Autodesk Inventor part; units mm, degrees
ref_plane "YZ Plane" through (0, 0, 0) normal (1, 0, 0) x (0, 1, 0)
ref_plane "XZ Plane" through (0, 0, 0) normal (0, 1, 0) x (-1, 0, 0)
ref_plane "XY Plane" through (0, 0, 0) normal (0, 0, 1) x (1, 0, 0)
sketch "Skizze1" plane through (0, 0, 0) normal (1, 0, 0) x (0, 1, 0)
  line L0 (0, 0) -> (-10, 0) construction
  circle A0 centre (0, 0) radius 1.1
  circle A1 centre (-10, 0) radius 1.1
  arc A2 (-10, 2.5) -> (-10, -2.5) centre (-10, 0) ccw
  line L1 (-10, -2.5) -> (1.8, -2.5)
  line L2 (-10, 2.5) -> (-0.7, 2.5)
  arc A3 (1.8, 0) -> (-0.7, 2.5) centre (-0.7, 0) ccw
  line L3 (1.8, 0) -> (1.8, -2.5)
  dimension "d0" = 10
  dimension "d1" = 2.2
  dimension "d2" = 2.2
  dimension "d3" = 2.5
  dimension "d8" = 2.5
  dimension "d9" = 1.8
extrude "Extrusion1" add sketch "Skizze1" along normal mid plane 4
chamfer "Fase1" distance 0.5 angle 45 10 edges at (2, 1.0678, 1.7678) (2, -5.35, 2.5) (2, -12.5, 0) (2, -4.1, -2.5) (2, 1.8, -1.25) (-2, 1.0678, 1.7678) (-2, -5.35, 2.5) (-2, -12.5, 0) (-2, -4.1, -2.5) (-2, 1.8, -1.25)
sketch "Skizze5" plane through (-1.5, -10, 2.5) normal (0, 0, 1) x (1, 0, 0)
  line L0 (1.5, 14.66) -> (1.5, -5.36)
  line L1 (-1.3, 10) -> (4.3, 10)
  line L2 (3.5, 8) -> (-0.5, 8)
  line L3 (-0.5, 8) -> (-0.5, 7)
  line L4 (-0.5, 7) -> (3.5, 7)
  line L5 (3.5, 7) -> (3.5, 8)
  line L6 (3.5, 0) -> (3.5, 9.3)
  line L7 (-0.5, 9.3) -> (-0.5, 0)
  point P0 (1.5, 10)
  dimension "d26" = 1
  dimension "d27" = 2
extrude "Extrusion4" cut sketch "Skizze5" against normal blind 1
equation "\"d2\" = d1"
properties part number "Chipanschlag TN1"
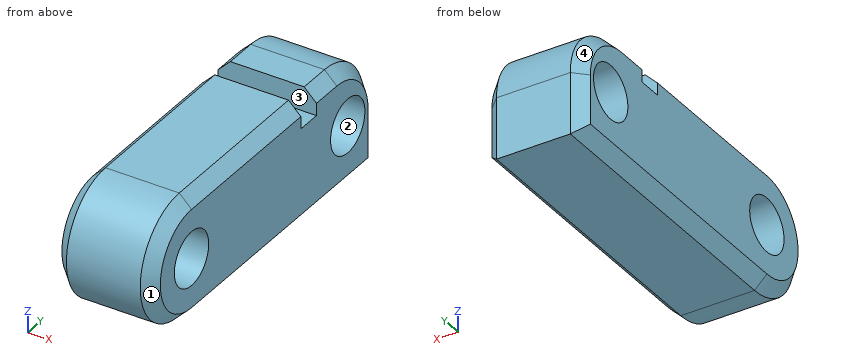
Part model, mm, in its own coordinate system. Face numbers are marked on the shaded views. Round coordinates to 2 decimals unless told otherwise and drop trailing zeros. Loops run counter-clockwise (first coordinate to the right, second up) from the corner with the lowest first, then second, coordinate; pieces in that order, holes last.
Item 1: Drop flat-ended pins along their axis: P1, Ø1.1, axis at x = 1, z = 2, coming from the -Y side; P2, Ø0.8, axis at x = -1, y = -2.5, coming from the +Z side. Give the stop position or say it passes through.
Item 2: Mould opens along Y. For the marked faces 1, 2, 3 and 4 say: +Y half, -Y half, draft (parallel to the pull), parting line (faces both ways), or undercut.
Item 3: Cut at A-A, the plane x = -1.65. Give the cut face in (y, z), then the cut area to 3 significant figures.
Item 4: Drill centre lines: line 1 (Z direction, x = 0.1, y = -10); line 2 (Y direction, x = -0.4, z = -0.8); line 3 (Z direction, x = -0.05, y = 0). Where is each one in solid material? Low to high.
Item 5: Cut at C-C, the plane z = -0.7. State how many separate pieces and enclosed holes the cut face has, then the cut area to 3 significant figures.
Item 6: Cut at B-B, the plane y = -7.75. Give the cut face in (x, z).
A:
1. P1: stops at y = -12.04
1. P2: stops at z = 1.5
2. face 1: -Y half
2. face 2: undercut
2. face 3: undercut
2. face 4: +Y half
3. outline: (-10, -2.35) - (1.65, -2.35) - (1.65, 0) arc R2.35 ccw to (-0.7, 2.35) - (-2, 2.35) - (-2, 1.5) - (-3, 1.5) - (-3, 2.35) - (-10, 2.35) arc R2.35 ccw to start; hole circle Ø2.2 at (-10, 0); hole circle Ø2.2 at (0, 0)
3. area: 53.8 mm2
4. line 1: z = -2.5 to -1.1, 1.1 to 2.5
4. line 2: y = -12.37 to -10.75, -9.25 to -0.75, 0.75 to 1.8
4. line 3: z = -2.5 to -1.1, 1.1 to 2.4
5. separate pieces: 3
5. enclosed holes: 0
5. area: 42.7 mm2
6. outline: (-2, -2) - (-1.5, -2.5) - (1.5, -2.5) - (2, -2) - (2, 2) - (1.5, 2.5) - (-1.5, 2.5) - (-2, 2) - close
